For this review, use the dimensioned drawing (mm, ordinates from the lowest corner) and the shaded views. Give positions to 0.01 mm unless a question says otherwise; leave off trailing zeros. Write each loop counter-clockwise with the first axis right and the second up, starting at its lowest first coordinate (ties: lowest second). Pieces come first, ordered by that corner, then holes. Notation, with made-up numbers: M 46,72 L 73,72 A20 ccw 73,107 Z; hole C -39.75,-3.5 d2. An arc over 180 degrees is marked long. One line per item, written item: value. Start each with the question number.
Item 1: Clearance check with flat-ended pins moving along their axes: pin 1 Ø3 at (y, z) = (2.5, 11) entering from +X; pin 2 Ø3 at (x, y) = (6, 2) entering from +Z; pin 3 Ø1 at (x, y) = (8.5, 1) entering from -Z; pin 4 Ø5 at (x, z) = (9, 9) entering from +Y. State where each tip first meets the part, or that it passes through.
Item 2: To check wall thickness, follow probe 1 along X at (y, z) = (3.2, 9); probe 2 along Z at (x, y) = (6, 2.6). State the ranges of each line that lie inside material, in increasing order.
Item 3: Mouldability with a two-part tool opening along Z and no side actions: class the marked faces 1, 2 and 3 as released by +Z, released by -Z, zero draft, split by the parting line, or undercut.
Item 4: Consider section B-B, the plane y = 3.5. Write out the cut boundary in (x, z).
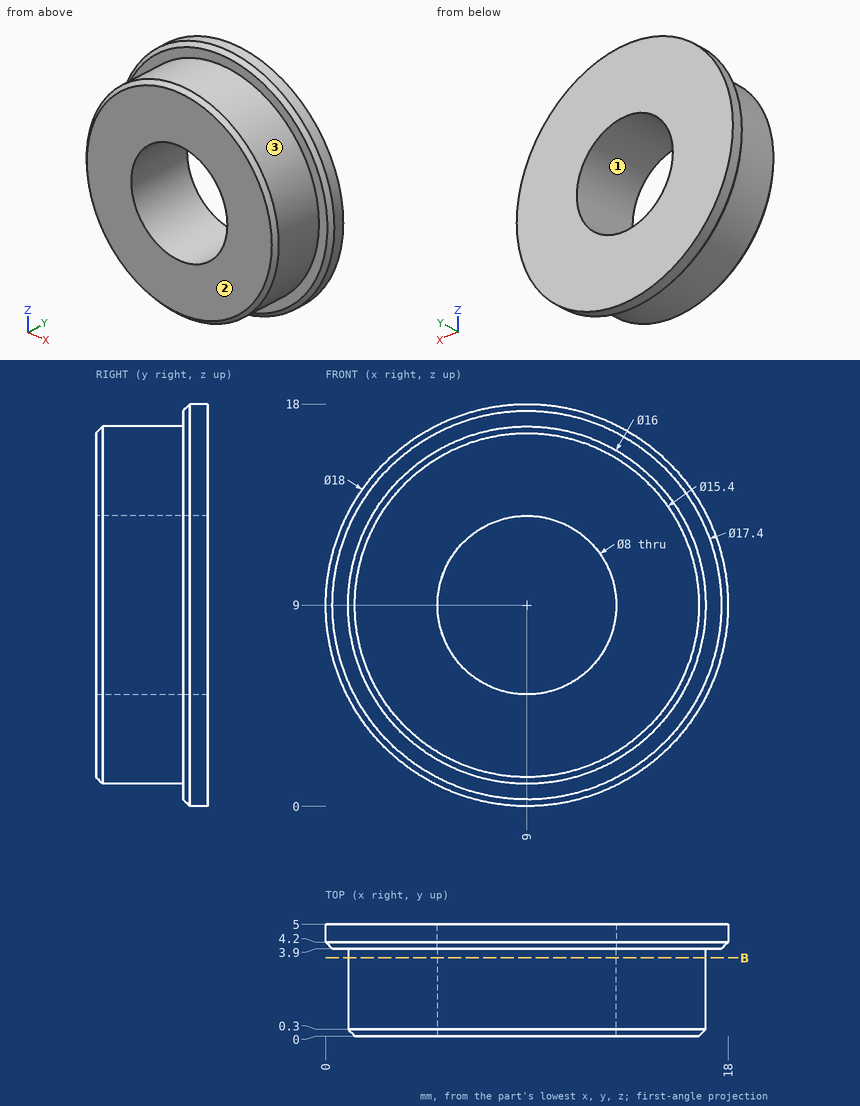
Model answer:
1. pin 1: stops at x = 17.6
1. pin 2: stops at z = 16.86
1. pin 3: stops at z = 1
1. pin 4: passes through
2. probe 1: x = 1 to 5, 13 to 17
2. probe 2: z = 1.58 to 6.35, 11.65 to 16.42
3. face 1: undercut
3. face 2: zero draft
3. face 3: split by the parting line
4. outline: C 9,9 d16; hole C 9,9 d8
